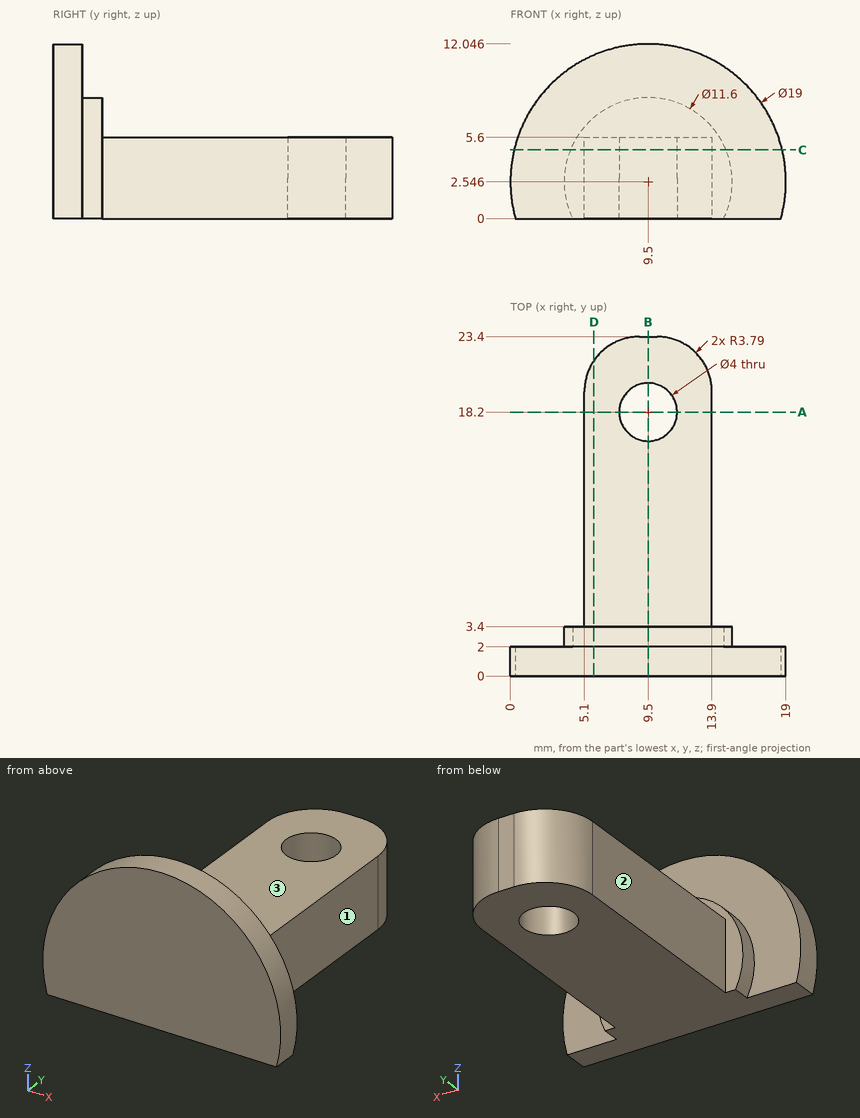
Design review of the part shown in the three views and the two pictorial views. Dimensions are in mm from the part's minimum x, y and z. A direction names the side the tool comes from. Give positions to 0.01 mm unless a question says otherwise; leave off trailing zeros. Write each loop counter-clockwise with the first axis right and the second up, starting at its lowest first coordinate (ties: lowest second). Pieces come first, ordered by that corner, then holes. Notation, with made-up numbers: M -24,-31.5 L -19,-31.5 A24 ccw -19,-20.5 Z; hole C 57.5,-26.75 d1. An arc over 180 degrees is marked long. Return JSON: item names as keys, results as strings. Group by question number.
Item 1: Take a section at B-B (x = 9.5). Give the boundary of the cut face in (y, z).
Item 2: Take a section at D-D (x = 5.75). Give the boundary of the cut face in (y, z), plus the area to 3 significant figures.
Item 3: Tool access review of the marked faces 1, 2 and 3: name each direction out of +Z, -Z, +X, -X, +Y, -Y from which nothing blocks a thin tool from reaching the whole face with its end or side.
Item 4: Clearance check with flat-ended pins moving along their axes: pin 1 Ø1 at (x, y) = (3.5, 19.5) entering from +Z; pin 2 Ø5 at (x, z) = (2.5, 5) entering from +Y; pin 3 Ø3 at (y, z) = (15, 3) entering from -X; pin 4 Ø5 at (y, z) = (11.5, 3.5) entering from +X. State where each tip first meets the part, or that it passes through.
Item 5: Take a section at A-A (y = 18.2). Give the boundary of the cut face in (x, z).
Item 6: Wall thickness on line 1 along Y through (x, z) = (9.5, 2); line 2 along Y through (x, z) = (16, 4); line 3 along Z through (x, y) = (12.75, 18.75): over which ranges is each line inside the solid? List them lowest first.
Item 7: Take a section at C-C (z = 4.75). Give the boundary of the cut face in (x, y) (1 decimal), plus the area to 3 significant figures.
Return value:
{
 "1": {"outline": "M 0,0 L 16.2,0 L 16.2,5.6 L 3.4,5.6 L 3.4,8.35 L 2,8.35 L 2,12.05 L 0,12.05 Z; M 20.2,0 L 23.4,0 L 23.4,5.6 L 20.2,5.6 Z"},
 "2": {"outline": "M 0,0 L 21.73,0 L 21.73,5.6 L 3.4,5.6 L 3.4,6.97 L 2,6.97 L 2,11.27 L 0,11.27 Z", "area": "135 mm2"},
 "3": {"face 1": "+Z, -Z, +X, +Y", "face 2": "+Z, -Z, -X, +Y", "face 3": "+Z, +X, -X, +Y"},
 "4": {"pin 1": "passes through", "pin 2": "stops at y = 3.4", "pin 3": "stops at x = 5.1", "pin 4": "stops at x = 13.9"},
 "5": {"outline": "M 5.1,0 L 7.5,0 L 7.5,5.6 L 5.1,5.6 Z; M 11.5,0 L 13.9,0 L 13.9,5.6 L 11.5,5.6 Z"},
 "6": {"line 1": "y = 0 to 16.2, 20.2 to 23.4", "line 2": "y = 0 to 2", "line 3": "z = 0 to 5.6"},
 "7": {"outline": "M 0.3,0 L 18.7,0 L 18.7,2 L 14.9,2 L 14.9,3.4 L 13.9,3.4 L 13.9,19.6 A3.8 ccw 10.1,23.4 L 8.9,23.4 A3.8 ccw 5.1,19.6 L 5.1,3.4 L 4.1,3.4 L 4.1,2 L 0.3,2 Z; hole C 9.5,18.2 d4", "area": "209 mm2"}
}
